Check sheet for the modelled part. Datum: model origin and axes. Units: mm. A direction names the side the tool comes from. Round coordinates to 2 decimals unless told otherwise and drop trailing zeros. Loops run counter-clockwise (first coordinate to the right, second up) from the corner with the lowest first, then second, coordinate; pieces in that order, holes last. Notation, with made-up numbers: M 37.25,6 L 87.25,6 A12 cw 87.25,14 Z; hole C -15,82.5 d3. An arc over 180 degrees is marked long. One line per question, with ' | ' between items. Start each with the question number.
(1) Tool access check on faces 1 (the face through (-4.829, 1.468, -1.915)), 2 (the face through (-11, 0, -1.588)), 3 (the face through (0, 0, 0)). Record the directions out of +Z, -Z, +X, -X, +Y, -Y that give a thin tool (end or side, any length) a straight path to the whole face; none if there is none.
(2) Thickness scan on probe 1 along X at (y, z) = (-3.5, 2.5); probe 2 along Y at (x, z) = (-1.75, 0.25); probe 3 along X at (y, z) = (-1.25, -4.25). Record the ranges inside material, lowest first. Write a range as [from, to].
(3) Section check B-B (x = -3.25). Record the boundary of the cut face in (y, z), and give its area (3 significant figures).
(4) Go/stop test with flat-tipped pins: P1, Ø4, axis at x = -1.5, y = -3.5, coming from the -Z side; P2, Ø1, axis at y = 0, z = -0.5, coming from the -X side; P3, Ø4, axis at x = -8, z = 1.5, coming from the +Y side. Record where each tip stops, or that it passes through.
```python
from build123d import *

# Parameters (mm, degrees)
CUT_EXTRUDE1_DEPTH = 2.54
FILLET1_R          = 0.0508


with BuildPart() as part:
    # Sketch1 → Revolve2 (revolve)
    with BuildSketch(Plane.XY, mode=Mode.PRIVATE) as revolve2_sk:
        Polygon((0, 0), (0, 2.413), (-9.525, 2.413), (-12.7, 5.2197), (-12.7, 0), align=None)
    revolve(revolve2_sk.sketch.rotate(Axis((-12.7, 0, 0), (1, 0, 0)), 90), axis=Axis((-12.7, 0, 0), (1, 0, 0)))

    # Sketch2 → Cut-Extrude1 (cut)
    with BuildSketch(Plane.ZY.offset(12.7)):
        Polygon((0, 1.833087105), (-1.5875, 0.916543552), (-1.5875, -0.916543552), (0, -1.833087105), (1.5875, -0.916543552), (1.5875, 0.916543552), align=None)
    extrude(amount=-CUT_EXTRUDE1_DEPTH, mode=Mode.SUBTRACT)

    # Fillet1
    fillet1_edges = [part.edges().sort_by_distance(p)[0] for p in [
        (-12.7, 1.374815329, 0.79375),
        (-12.7, 1.374815329, -0.79375),
        (-12.7, 0, -1.5875),
        (-12.7, -1.374815329, -0.79375),
        (-12.7, -1.374815329, 0.79375),
        (-12.7, 0, 1.5875),
    ]]
    fillet(fillet1_edges, radius=FILLET1_R)


solid = part.part
```
The answers:
1) face 1: +X | face 2: -X | face 3: +Z, -Z, +X, +Y, -Y
2) probe 1: [-12.7, -11.66] | probe 2: [-2.4, 2.4] | probe 3: [-12.7, -11.81]
3) outline: C 0,0 d4.83 | area: 18.3 mm²
4) P1: z = -1.89 | P2: x = -10.16 | P3: y = 2.6
